Work out the finished part from the listing and answer in its coordinate system (mm). A direction names the side the tool comes from. Coordinates: 2 decimals unless noted, no trailing zeros. Order: outer loops, then holes, each group sorted by start corner. A loop starts at its lowest first (then second) coordinate and runs counter-clockwise, first axis right, second up. Notation, with made-up numbers: M -14,76.5 L -5,76.5 A19 ccw -5,103.5 Z; hole C -21,85 d6. An arc over 180 degrees is marked long. Use a Markdown table: item, result.
from build123d import *

# Parameters (mm, degrees)
F0_R     = 1.6
F0_W     = 11.2395305085
F0_H     = 70
F0_W_2   = 89.7604694915
F0_W_3   = 6.7604694915
F1_DEPTH = 3.175


# Not quite as in the source:
# - a length typed as a fraction of an inch, garbled in the dataset ("3 / 203.2 mm" for 3/8 in), is restored


with BuildPart() as f1:
    # F0 (on Front) → F1 (new body)
    with BuildSketch(Plane.XZ):
        with BuildLine():
            Line((21.2395305085, 0), (6.35, 0))
            ThreePointArc((6.35, 0), (1.8598719395, -1.8598719395), (0, -6.35))
            Line((0, -6.35), (0, -83.65))
            ThreePointArc((0, -83.65), (1.8598719395, -88.1401280605), (6.35, -90))
            Line((6.35, -90), (21.2395305085, -90))
            Line((21.2395305085, -90), (31.2395305085, -90))
            Line((31.2395305085, -90), (143.65, -90))
            ThreePointArc((143.65, -90), (148.1401280605, -88.1401280605), (150, -83.65))
            Line((150, -83.65), (150, -6.35))
            ThreePointArc((150, -6.35), (148.1401280605, -1.8598719395), (143.65, 0))
            Line((143.65, 0), (31.2395305085, 0))
            Line((31.2395305085, 0), (21.2395305085, 0))
        make_face()
        with Locations((75, -85)):
            Circle(F0_R, mode=Mode.SUBTRACT)
        with Locations((15.6197652543, -45)):
            Rectangle(F0_W, F0_H, mode=Mode.SUBTRACT)
        with Locations((26.162, -14.986)):
            Circle(F0_R, mode=Mode.SUBTRACT)
        with Locations((26.2395305085, -5)):
            Circle(F0_R, mode=Mode.SUBTRACT)
        with Locations((52.9, -5)):
            Circle(F0_R, mode=Mode.SUBTRACT)
        with Locations((76.1197652543, -45)):
            Rectangle(F0_W_2, F0_H, mode=Mode.SUBTRACT)
        with Locations((136.6197652543, -45)):
            Rectangle(F0_W_3, F0_H, mode=Mode.SUBTRACT)
        with Locations((97.1, -5)):
            Circle(F0_R, mode=Mode.SUBTRACT)
    extrude(amount=F1_DEPTH)


solid = f1.part
1. For faces 4 (the face through (148.09, -1.57, -88.19)), 5 (the face through (137, -2, -10)), determine the directions among +Z, -Z, +X, -X, +Y, -Y from which every point of the face is accessible in a straight line to the end or side of a thin tool.
Answers below:
| item | result |
|---|---|
| face 4 | -Z, +X, +Y, -Y |
| face 5 | +Y, -Y |
2. Section A-A on x = 75 is taken. Determine the outline of the cut face in (y, z) (3 decimals), then the cut area to 3 significant figures.
Answers below:
| item | result |
|---|---|
| outline | M -3.175,-90 L 0,-90 L 0,-86.6 L -3.175,-86.6 Z; M -3.175,-83.4 L 0,-83.4 L 0,-80 L -3.175,-80 Z; M -3.175,-10 L 0,-10 L 0,0 L -3.175,0 Z |
| area | 53.3 mm² |
3. Find the intervals of material crossed by probe 1 along Z at (x, y) = (52.9, -2.4); probe 2 along X at (y, z) = (-2.35, -67.5); probe 3 along Z at (x, y) = (120.5, -1.65), in increasing order.
Answers below:
| item | result |
|---|---|
| probe 1 | -90 to -80, -10 to -6.6, -3.4 to 0 |
| probe 2 | 0 to 10, 21.24 to 31.24, 121 to 133.24, 140 to 150 |
| probe 3 | -90 to -80, -10 to 0 |
4. A flat-ended cylindrical pin translates along its axis: P1, Ø8, axis at x = 48, z = -73.5, coming from the +Y side. Find the tip coordinate at first contact, or state that the pin passes through.
Answers below:
| item | result |
|---|---|
| P1 | through |
5. Section B-B on z = -64.5 is taken. Determine the outline of the cut face in (x, y) (3 decimals).
Answers below:
| item | result |
|---|---|
| outline | M 0,-3.175 L 10,-3.175 L 10,0 L 0,0 Z; M 21.24,-3.175 L 31.24,-3.175 L 31.24,0 L 21.24,0 Z; M 121,-3.175 L 133.24,-3.175 L 133.24,0 L 121,0 Z; M 140,-3.175 L 150,-3.175 L 150,0 L 140,0 Z |
6. For a pull along Z with two mould halves and no side action, classify faces 1 (the face through (21.24, -2, -45)), 2 (the face through (74, -3.175, -4)), 3 (the face through (148.19, -1.57, -1.91)) as +Z half, -Z half, draft (parallel to the pull), parting line (faces both ways), or undercut.
Answers below:
| item | result |
|---|---|
| face 1 | undercut |
| face 2 | draft |
| face 3 | +Z half |
7. Section C-C on y = -1.7 is taken. Give the number of separate pieces and of enclosed holes in the cut face, then the cut area to 3 significant figures.
Answers below:
| item | result |
|---|---|
| separate pieces | 1 |
| enclosed holes | 8 |
| area | 5,880 mm² |
